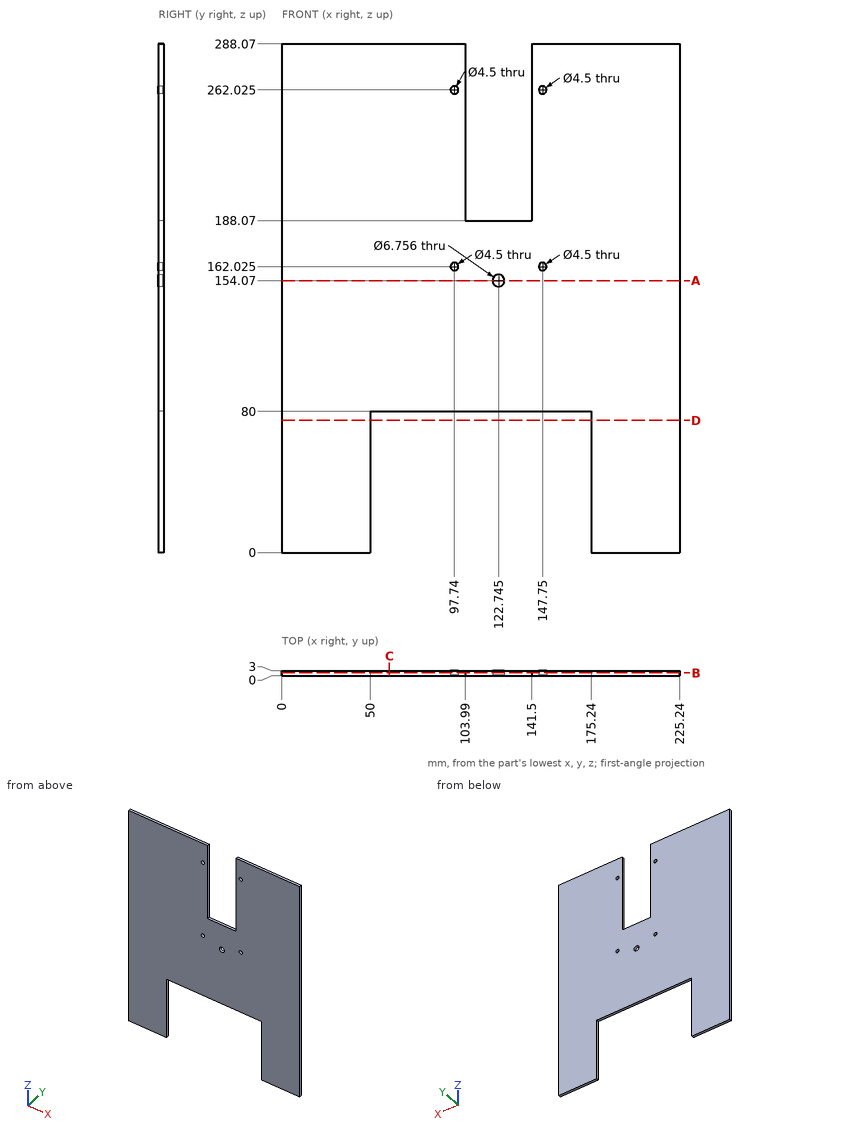
Part print with two shaded views. Sizes in mm from the minimum x, y, z corner. Round coordinates to 2 decimals unless told otherwise and drop trailing zeros. Write each loop counter-clockwise with the first axis right and the second up, starting at its lowest first coordinate (ties: lowest second). Pieces come first, ordered by that corner, then holes. Notation, with made-up numbers: (78.5, 61) -> (123.5, 61) arc R15 cw to (123.5, 84) -> close; hole circle Ø2 at (13, 88.5). An arc over 180 degrees is marked (long way). Put each result on its own line as item: value.
Item 1: Wall check: probe 1 along Z at (x, y) = (147.75, 2.3) (1 decimal); probe 2 along X at (y, z) = (1.3, 188.5); probe 3 along X at (y, z) = (1.45, 67). Give the ranges that are in metal, low to high. Write a range as from..to.
Here are the results:
probe 1: z = 80..159.8, 164.3..259.8, 264.3..288.1
probe 2: x = 0..103.99, 141.5..225.24
probe 3: x = 0..50, 175.24..225.24
Item 2: Flat gauge pins, fed straight in: P1, Ø8, axis at x = 153.5, z = 248, coming from the -Y side; P2, Ø1.5, axis at x = 91.5, y = 2, coming from the -Z side. Where does each tip first touch, or does it go through?
Here are the results:
P1: stops at y = 0
P2: stops at z = 80
Item 3: Slice it at B-B, the plane y = 1.75. Count the separate pieces of the cut face and the enclosed holes in it, plus the area to 3 significant figures.
Here are the results:
separate pieces: 1
enclosed holes: 5
area: 51,000 mm^2
Item 4: Slice it at D-D, the plane z = 75. Give the cut face in (x, y).
Here are the results:
outline: (0, 0) -> (50, 0) -> (50, 3) -> (0, 3) -> close; (175.24, 0) -> (225.24, 0) -> (225.24, 3) -> (175.24, 3) -> close
Item 5: Slice it at C-C, the plane x = 61. Give the cut face in (y, z).
Here are the results:
outline: (0, 80) -> (3, 80) -> (3, 288.07) -> (0, 288.07) -> close
Item 6: Slice it at A-A, the plane z = 154.07. Give the cut face in (x, y).
Here are the results:
outline: (0, 0) -> (119.37, 0) -> (119.37, 3) -> (0, 3) -> close; (126.12, 0) -> (225.24, 0) -> (225.24, 3) -> (126.12, 3) -> close
